```python
from build123d import *

# Parameters (mm, degrees)
ESBO_O2_R                = 10.4
RESSALTO_EXTRUS_O1_DEPTH = 7.5
CORTE_EXTRUS_O1_DEPTH    = 17.509694122
PADR_OCIRCULAR2_COUNT    = 8
ESBO_O3_R                = 6
RESSALTO_EXTRUS_O2_DEPTH = 20


with BuildPart() as part:
    # Esboço2 → Ressalto-extrusão1 (new body)
    with BuildSketch(Plane.XY):
        Circle(ESBO_O2_R)
    extrude(amount=RESSALTO_EXTRUS_O1_DEPTH)

    # Esboço1 → Corte-extrusão1 (cut, through all)
    with BuildSketch(Plane.XY):
        with BuildLine():
            Line((-0.506751832, 5.642289215), (-1.097919721, 7.266509641))
            ThreePointArc((-1.097919721, 7.266509641), (-1.406126414, 7.910707201), (-1.832951119, 8.483247621))
            ThreePointArc((-1.832951119, 8.483247621), (-2.661618953, 9.214061597), (-3.630088541, 9.745894376))
            ThreePointArc((-3.630088541, 9.745894376), (0, 10.4), (3.630088541, 9.745894376))
            ThreePointArc((3.630088541, 9.745894376), (2.661618953, 9.214061597), (1.832951119, 8.483247621))
            ThreePointArc((1.832951119, 8.483247621), (1.406126414, 7.910707201), (1.097919721, 7.266509641))
            Line((1.097919721, 7.266509641), (0.506751832, 5.642289215))
            ThreePointArc((0.506751832, 5.642289215), (0, 5.665), (-0.506751832, 5.642289215))
        make_face()
    corte_extrus_o1 = extrude(amount=CORTE_EXTRUS_O1_DEPTH, mode=Mode.SUBTRACT)

    # PadrãoCircular2: Corte-extrusão1 ×8 about axis
    padr_ocircular2_axis = Axis((0, 0, 0), (0, 0, 1))
    for i in range(1, PADR_OCIRCULAR2_COUNT):
        add(corte_extrus_o1.rotate(padr_ocircular2_axis, i * 360 / PADR_OCIRCULAR2_COUNT), mode=Mode.SUBTRACT)

    # Esboço3 → Ressalto-extrusão2 (add)
    with BuildSketch(Plane(origin=(0, 0, 0), x_dir=(-1, 0, 0), z_dir=(0, 0, -1))):
        with Locations(Location((0, 0, 0), (0, 0, 174.020217927))):
            Circle(ESBO_O3_R)
    extrude(amount=RESSALTO_EXTRUS_O2_DEPTH)


solid = part.part
```
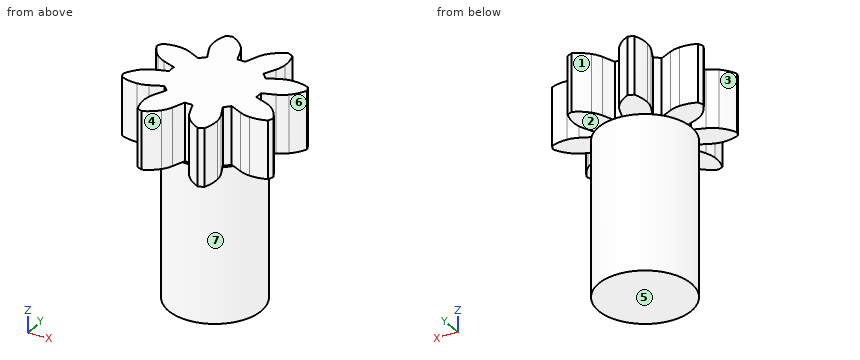
Part model, mm, in its own coordinate system. Face numbers are marked on the shaded views. A direction names the side the tool comes from. Give positions to 0.01 mm unless a question says otherwise; leave off trailing zeros. Write each loop counter-clockwise with the first axis right and the second up, starting at its lowest first coordinate (ties: lowest second). Pieces come first, ordered by that corner, then holes. Notation, with made-up numbers: (61.5, 39) -> (72.5, 39) arc R28 ccw to (72.5, 62) -> close; hole circle Ø4 at (33, 12). An arc over 180 degrees is marked (long way). Put each result on its own line as item: value. Start each with the question number.
Item 1: Cut at B-B (y = 0). List the corners of the cut face in (x, z) (3 decimals).
Item 2: Cut at D-D (x = -6.75). List the corners of the cut face in (y, z).
Item 3: Pin check, flat tips, straight feed: pin 1 Ø3.5 at (x, y) = (2.5, -7.5) entering from -Z; pin 2 Ø6 at (x, z) = (-6, -8.5) entering from -Y; pin 3 Ø1 at (x, z) = (-4.5, -4) entering from -Y. Stop position of each tip, or through.
Item 4: Cut at A-A (x = 7.75). List the corners of the cut face in (y, z).
Item 5: Cut at C-C (x = 2.5). List the corners of the cut face in (y, z).
Item 6: Pull direction X, two halves, no side cores. Call the marked faces 1, 2, 3 and 4: pulls with the +X half, pulls with the -X half, needs draft (parallel to the pull), parting line crosses it, or undercut.
Item 7: Which spindle directions (+Z, -Z, +X, -X, +Y, -Y) get a long thin tool onto all of the face, cutting with end or side? Do the marked faces 5, 6 and 7. Say none if no direction does.
Item 8: Wall check: L1, parallel to Z at x = 7.25, y = 2.5; L2, parallel to X at y = 1, z = -0.5; L3, parallel to X at y = 0, z = -15.5. Give the ranges that are in metal, low to high. Write a range as [from, to].
Answer list:
1. outline: (-6, -20) -> (6, -20) -> (6, 0) -> (5.665, 0) -> (5.665, 7.5) -> (-5.665, 7.5) -> (-5.665, 0) -> (-6, 0) -> close
2. outline: (-4.64, 0) -> (-0.91, 0) -> (-0.91, 7.5) -> (-4.64, 7.5) -> close; (0.91, 0) -> (4.64, 0) -> (4.64, 7.5) -> (0.91, 7.5) -> close
3. pin 1: stops at z = 0
3. pin 2: stops at y = -5.2
3. pin 3: stops at y = -4.47
4. outline: (-4.7, 0) -> (-1.31, 0) -> (-1.31, 7.5) -> (-4.7, 7.5) -> close; (1.31, 0) -> (4.7, 0) -> (4.7, 7.5) -> (1.31, 7.5) -> close
5. outline: (-9.1, 0) -> (-5.45, 0) -> (-5.45, -20) -> (5.45, -20) -> (5.45, 0) -> (9.1, 0) -> (9.1, 7.5) -> (-9.1, 7.5) -> close
6. face 1: undercut
6. face 2: needs draft
6. face 3: pulls with the -X half
6. face 4: undercut
7. face 5: -Z, +X, -X, +Y, -Y
7. face 6: +Z, -Z, +X
7. face 7: -Z
8. L1: z = [0, 7.5]
8. L2: x = [-5.92, 5.92]
8. L3: x = [-6, 6]
